Autodesk Inventor part; units mm, degrees
ref_plane "YZ Plane" through (0, 0, 0) normal (1, 0, 0) x (0, 1, 0)
ref_plane "XZ Plane" through (0, 0, 0) normal (0, 1, 0) x (-1, 0, 0)
ref_plane "XY Plane" through (0, 0, 0) normal (0, 0, 1) x (1, 0, 0)
sketch "Sketch1" plane through (0, 0, 0) normal (0, 0, 1) x (1, 0, 0)
  line L0 (0, 0) -> (64.8574, 0) construction
  line L1 (-30, -55) -> (30, -55)
  line L2 (30, -55) -> (30, 55)
  line L3 (30, 55) -> (-30, 55)
  line L4 (-30, 55) -> (-30, -55)
  line L5 (-30, -55) -> (30, 55) construction
  line L6 (30, -55) -> (-30, 55) construction
  dimension "d0" = 60
  dimension "d1" = 110
extrude "Extrusion1" add sketch "Sketch1" along normal blind 3
fillet "Fillet1" radius 10.25 4 edges at (30, 55, 1.5) (-30, 55, 1.5) (30, -55, 1.5) (-30, -55, 1.5)
sketch "Sketch2" plane through (0, 0, 3) normal (0, 0, 1) x (1, 0, 0)
  line L0 (0, 0) -> (47.0336, 0) construction
  line L1 (-30, -55) -> (30, -55)
  line L2 (30, -55) -> (30, 55)
  line L3 (30, 55) -> (-30, 55)
  line L4 (-30, 55) -> (-30, -55)
  line L5 (-30, -55) -> (30, 55) construction
  line L6 (30, -55) -> (-30, 55) construction
  line L7 (-28.5, 53.5) -> (28.5, 53.5)
  line L8 (28.5, 53.5) -> (28.5, -53.5)
  line L9 (28.5, -53.5) -> (-28.5, -53.5)
  line L10 (-28.5, -53.5) -> (-28.5, 53.5)
  dimension "d5" = 60
  dimension "d6" = 110
  dimension "d7" = 1.5
extrude "Extrusion2" add sketch "Sketch2" along normal blind 2 contours L7 L8 L9 L10
fillet "Fillet2" radius 10.25 4 edges at (28.5, 53.5, 4) (-28.5, 53.5, 4) (-28.5, -53.5, 4) (28.5, -53.5, 4)
sketch "Sketch3" plane through (0, 0, 0) normal (0, 0, -1) x (-1, 0, 0)
  line L0 (9, 43.8265) -> (-9, 43.8265) construction
  line L1 (9, 45.3265) -> (-9, 45.3265)
  line L2 (-9, 42.3265) -> (9, 42.3265)
  arc A0 (9, 42.3265) -> (9, 45.3265) centre (9, 43.8265) ccw
  arc A1 (-9, 45.3265) -> (-9, 42.3265) centre (-9, 43.8265) ccw
  line L3 (-9, 46.8265) -> (9, 46.8265)
  arc A2 (9, 40.8265) -> (9, 46.8265) centre (9, 43.8265) ccw
  line L4 (9, 40.8265) -> (-9, 40.8265)
  arc A3 (-9, 46.8265) -> (-9, 40.8265) centre (-9, 43.8265) ccw
  point P0 (0, 0)
  point P1 (0, 43.8265)
  dimension "d11" = 9
  dimension "d12" = 3
  dimension "d15" = 1.5
extrude "Extrusion3" cut sketch "Sketch3" against normal through all contours A0 L2 A1 L1 | L3 A2 L4 A3
sketch "Sketch4" plane through (0, 0, 4) normal (0, 0, -1) x (-1, 0, 0)
  point P0 (0, 0)
properties part number "BackPlate"
Input: part model. Units: mm. Frame: model coordinates. A direction names the side the tool comes from. Coordinates: 2 decimals unless noted, no trailing zeros. Loops run counter-clockwise (first coordinate to the right, second up) from the corner with the lowest first, then second, coordinate; pieces in that order, holes last. Notation, with made-up numbers: (-36, -1.5) -> (13, -1.5) arc R15 cw to (13, 16.5) -> close; hole circle Ø8 at (78.5, 49.25). An arc over 180 degrees is marked (long way). One line per item, written item: value.
(1) Set-up query: faces 4 (the face through (-28.5, -1, 4)), 5 (the face through (25.418, 50.577, 3.986)), 6 (the face through (12, 43.9, 2.5)), 7 (the face through (28.5, 1, 4)), 8 (the face through (0, 53.5, 4)). Return all of +Z, -Z, +X, -X, +Y, -Y with unobstructed straight access to the full face (end or side cutting, diameter ignored); none if empty.
Answer below:
face 4: +Z, -X, +Y, -Y
face 5: +Z, +X, +Y
face 6: +Z, -Z
face 7: +Z, +X, +Y, -Y
face 8: +Z, +X, -X, +Y
(2) Ray query, line 1 along X through (y, z) = (12.5, 3.05); line 2 along Y through (x, z) = (-6, 1.3); line 3 along Y through (x, z) = (-9.5, 0.8). Return the intervals inside material, ascending.
Answer below:
line 1: x = -28.5 to 28.5
line 2: y = -55 to 40.83, 46.83 to 55
line 3: y = -55 to 40.87, 46.78 to 55
(3) Pin query (flat end, axial travel): pin 1 Ø1.6 at (x, z) = (4.5, 4) entering from -Y; pin 2 Ø1.6 at (y, z) = (2.5, 4) entering from -X; pin 3 Ø0.6 at (x, z) = (0.5, 3.5) entering from +Y. Return the tip coordinate at first contact, or that it passes through.
Answer below:
pin 1: stops at y = -53.5
pin 2: stops at x = -28.5
pin 3: stops at y = 53.5
(4) Cut plane B-B (y = 38). Output: boundary loops of the cut face in (x, z).
Answer below:
outline: (-30, 0) -> (30, 0) -> (30, 3) -> (28.5, 3) -> (28.5, 5) -> (-28.5, 5) -> (-28.5, 3) -> (-30, 3) -> close
(5) Cut plane C-C (x = 24.5). Output: boundary loops of the cut face in (y, z).
Answer below:
outline: (-53.83, 0) -> (53.83, 0) -> (53.83, 3) -> (51.37, 3) -> (51.37, 5) -> (-51.37, 5) -> (-51.37, 3) -> (-53.83, 3) -> close
(6) Draft query along Y for faces 1 (the face through (-12, 43.8, 2.5)), 2 (the face through (-29, 0, 3)), 3 (the face through (0, -53.5, 4)). Return one class per face: pulls with the +Y half, pulls with the -Y half, needs draft (parallel to the pull), parting line crosses it, or undercut.
Answer below:
face 1: undercut
face 2: needs draft
face 3: pulls with the -Y half
(7) Cut plane A-A (z = 3.8). Output: boundary loops of the cut face in (x, y), then the cut area to 3 significant figures.
Answer below:
outline: (-28.5, -43.25) arc R10.25 ccw to (-18.25, -53.5) -> (18.25, -53.5) arc R10.25 ccw to (28.5, -43.25) -> (28.5, 43.25) arc R10.25 ccw to (18.25, 53.5) -> (-18.25, 53.5) arc R10.25 ccw to (-28.5, 43.25) -> close; hole (-9, 40.83) -> (9, 40.83) arc R3 ccw to (9, 46.83) -> (-9, 46.83) arc R3 ccw to start
area: 5,870 mm2
